For this review, take the finished solid that the model builds, in its own axes (mm). Coordinates: 2 decimals unless noted, no trailing zeros. Loops run counter-clockwise (first coordinate to the right, second up) from the corner with the lowest first, then second, coordinate; pieces in that order, holes last. Notation, with made-up numbers: (71, 24.5) -> (122, 24.5) arc R26 ccw to (122, 42.5) -> close; hole circle Ø8 at (56, -17). An arc over 180 degrees is marked (long way). Answer in a Markdown table with one row per item.
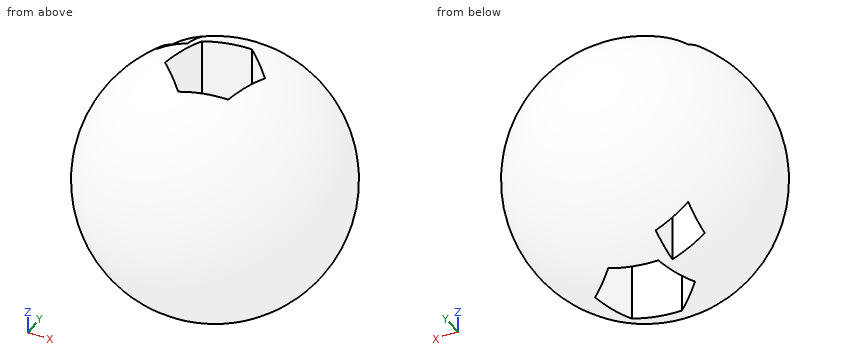
from build123d import *

# Parameters (mm, degrees)
F2_W     = 14.282297
F2_H     = 13.699342
F3_DEPTH = 67.818
F4_DEPTH = 221.996
F6_DEPTH = 96.774
F7_DEPTH = 104.648


with BuildPart() as f1:
    # F0 (on Front) → F1 (revolve)
    with BuildSketch(Plane.XZ):
        with BuildLine():
            Line((0, -55.817544), (0, 55.817544))
            ThreePointArc((0, 55.817544), (-55.817544, 0), (0, -55.817544))
        make_face()
    revolve(axis=Axis((0, 0, 0.145737), (0, 0, -1)))

    # F2 (on Top) → F3 (cut)
    with BuildSketch(Plane.XY):
        with Locations((-25.504099, 18.654426)):
            Rectangle(F2_W, F2_H)
    extrude(amount=-F3_DEPTH, mode=Mode.SUBTRACT)

    # F2 (on Top) → F4 (cut)
    with BuildSketch(Plane.XY):
        with Locations((-25.504099, 18.654426)):
            Rectangle(F2_W, F2_H)
    extrude(amount=F4_DEPTH, mode=Mode.SUBTRACT)

    # F5 (on Top) → F6 (cut)
    with BuildSketch(Plane.XY):
        Polygon((19.57916, 4.506355), (5.886962, 19.209227), (-13.692198, 14.702872), (-19.57916, -4.506355), (-5.886962, -19.209227), (13.692198, -14.702872), align=None)
    extrude(amount=-F6_DEPTH, mode=Mode.SUBTRACT)

    # F6_face (on face) → F7 (cut)
    with BuildSketch(Plane(origin=(0, 0, 0), x_dir=(1, 0, 0), z_dir=(0, 0, -1))):
        Polygon((5.886962, -19.209227), (19.57916, -4.506355), (13.692198, 14.702872), (-5.886962, 19.209227), (-19.57916, 4.506355), (-13.692198, -14.702872), align=None)
    extrude(amount=-F7_DEPTH, mode=Mode.SUBTRACT)


solid = f1.part
Item 1: Take a section at C-C, the plane x = 31. State the section outline as (y, z) points.
Worked answers:
| item | result |
|---|---|
| outline | circle Ø92.84 at (0, 0) |
Item 2: Take a section at A-A, the plane z = -41. State the section outline as (x, y) points.
Worked answers:
| item | result |
|---|---|
| outline | (-32.65, 11.8) -> (-32.65, 19.21) arc R37.88 ccw (long way) to (-28, 25.5) -> (-18.36, 25.5) -> (-18.36, 11.8) -> close; hole (-19.58, -4.51) -> (-5.89, -19.21) -> (13.69, -14.7) -> (19.58, 4.51) -> (5.89, 19.21) -> (-13.69, 14.7) -> close |
Item 3: For L1, parallel to X at y = 1, z = 38; L2, parallel to Y at x = -22.5, z = 36; L3, parallel to X at y = -39, z = 35, list the stretches that pass through material, from the lowest coordinate up.
Worked answers:
| item | result |
|---|---|
| L1 | -40.87 to -17.89, 18.5 to 40.87 |
| L2 | -36.24 to 11.8, 25.5 to 36.24 |
| L3 | -19.22 to 19.22 |
Item 4: Take a section at B-B, the plane z = -18. State the section outline as (x, y) points, and give its area (3 significant figures).
Worked answers:
| item | result |
|---|---|
| outline | circle Ø105.67 at (0, 0); hole (-32.65, 11.8) -> (-18.36, 11.8) -> (-18.36, 25.5) -> (-32.65, 25.5) -> close; hole (-19.58, -4.51) -> (-5.89, -19.21) -> (13.69, -14.7) -> (19.58, 4.51) -> (5.89, 19.21) -> (-13.69, 14.7) -> close |
| area | 7,530 mm² |
Item 5: Take a section at D-D, the plane y = 47.5. State the section outline as (x, z) points, and give its area (3 significant figures).
Worked answers:
| item | result |
|---|---|
| outline | circle Ø58.63 at (0, 0) |
| area | 2,700 mm² |
Item 6: Insertion check: pin 1 (1.5 mm diameter, centred on x = -32.5, y = -17.5, fed in from +Z); pin 2 (12 mm diameter, centred on y = 15.5, z = -22.5, fed in from -X); pin 3 (4 mm diameter, centred on y = 21, z = -20.5, fed in from +X). Each pin has a flat end and moves straight along its axis. Give the tip position at first contact, or say it passes through.
Worked answers:
| item | result |
|---|---|
| pin 1 | z = 42.52 |
| pin 2 | x = -51.58 |
| pin 3 | x = 48.66 |
